from build123d import *

# Parameters (mm, degrees)
ESQUISSE1_R                  = 5.75
ESQUISSE1_R_2                = 1.6
BOSS_EXTRU_1_DEPTH           = 5
ESQUISSE2_R                  = 3
ENL_V_MAT_EXTRU_1_DEPTH      = 3
ENL_V_START                  = -3
ESQUISSE3_R                  = 5.75
ESQUISSE3_R_2                = 4.5
ENL_V_MAT_EXTRU_2_DEPTH      = 3
BOSS_EXTRU_2_DEPTH           = 2
R_P_TITION_CIRCULAIRE1_COUNT = 2
ESQUISSE5_R                  = 0.75
ENL_V_MAT_EXTRU_3_DEPTH      = 3
R_P_TITION_CIRCULAIRE2_COUNT = 2
BOSS_EXTRU_3_DEPTH           = 3
R_P_TITION_CIRCULAIRE3_COUNT = 28
ENL_V_START_2                = -1
ESQUISSE7_R                  = 3
ESQUISSE7_R_2                = 1.6
ENL_V_MAT_EXTRU_4_DEPTH      = 1
ESQUISSE8_R                  = 4.7
ESQUISSE8_R_2                = 3.4
ENL_V_MAT_EXTRU_5_DEPTH      = 1
WYTNIJ_WYCI_GNI_CIE1_DEPTH   = 10


with BuildPart() as part:
    # Esquisse1 → Boss.-Extru.1 (new body)
    with BuildSketch(Plane.XY):
        Circle(ESQUISSE1_R)
        Circle(ESQUISSE1_R_2, mode=Mode.SUBTRACT)
    extrude(amount=BOSS_EXTRU_1_DEPTH)

    # Esquisse2 → Enlèv. mat.-Extru.1 (cut)
    with BuildSketch(Plane.XY.offset(5)):
        Circle(ESQUISSE2_R)
    extrude(amount=-ENL_V_MAT_EXTRU_1_DEPTH, mode=Mode.SUBTRACT)

    # Esquisse3 → Enlèv. mat.-Extru.2 (cut)
    with BuildSketch(Plane.XY.offset(5).offset(ENL_V_START)):
        Circle(ESQUISSE3_R)
        Circle(ESQUISSE3_R_2, mode=Mode.SUBTRACT)
    extrude(amount=ENL_V_MAT_EXTRU_2_DEPTH, mode=Mode.SUBTRACT)

    # Esquisse4 → Boss.-Extru.2 (add)
    with BuildSketch(Plane(origin=(0, 0, 0), x_dir=(-1, 0, 0), z_dir=(0, 0, -1))):
        with BuildLine():
            Line((-4.3, 3.817394399), (-2.475852955, 16.846629695))
            ThreePointArc((-2.475852955, 16.846629695), (0, 19), (2.475852955, 16.846629695))
            Line((2.475852955, 16.846629695), (4.3, 3.817394399))
            ThreePointArc((4.3, 3.817394399), (0, 5.75), (-4.3, 3.817394399))
        make_face()
    boss_extru_2 = extrude(amount=-BOSS_EXTRU_2_DEPTH)

    # Répétition circulaire1: Boss.-Extru.2 ×2 about axis
    r_p_tition_circulaire1_axis = Axis((0, 0, 0), (0, 0, 1))
    for i in range(1, R_P_TITION_CIRCULAIRE1_COUNT):
        add(boss_extru_2.rotate(r_p_tition_circulaire1_axis, i * 360 / R_P_TITION_CIRCULAIRE1_COUNT))

    # Esquisse5 → Enlèv. mat.-Extru.3 (cut)
    with BuildSketch(Plane(origin=(0, 0, 0), x_dir=(-1, 0, 0), z_dir=(0, 0, -1))):
        with Locations((0, 7)):
            Circle(ESQUISSE5_R)
        with Locations((0, 10)):
            Circle(ESQUISSE5_R)
        with Locations((0, 13)):
            Circle(ESQUISSE5_R)
        with Locations((0, 16)):
            Circle(ESQUISSE5_R)
    enl_v_mat_extru_3 = extrude(amount=-ENL_V_MAT_EXTRU_3_DEPTH, mode=Mode.SUBTRACT)

    # Répétition circulaire2: Enlèv. mat.-Extru.3 ×2 about axis
    r_p_tition_circulaire2_axis = Axis((0, 0, 0), (0, 0, 1))
    for i in range(1, R_P_TITION_CIRCULAIRE2_COUNT):
        add(enl_v_mat_extru_3.rotate(r_p_tition_circulaire2_axis, i * 360 / R_P_TITION_CIRCULAIRE2_COUNT), mode=Mode.SUBTRACT)

    # Esquisse6 → Boss.-Extru.3 (add)
    with BuildSketch(Plane.XY.offset(5)):
        Polygon((-0.3, 3), (0, 2.7), (0.3, 3), align=None)
    boss_extru_3 = extrude(amount=-BOSS_EXTRU_3_DEPTH)

    # Répétition circulaire3: Boss.-Extru.3 ×28 about axis
    r_p_tition_circulaire3_axis = Axis((0, 0, 0), (0, 0, 1))
    for i in range(1, R_P_TITION_CIRCULAIRE3_COUNT):
        add(boss_extru_3.rotate(r_p_tition_circulaire3_axis, i * 360 / R_P_TITION_CIRCULAIRE3_COUNT))

    # Esquisse7 → Enlèv. mat.-Extru.4 (cut)
    with BuildSketch(Plane(origin=(0, 0, 0), x_dir=(-1, 0, 0), z_dir=(0, 0, -1)).offset(ENL_V_START_2)):
        Circle(ESQUISSE7_R)
        Circle(ESQUISSE7_R_2, mode=Mode.SUBTRACT)
    extrude(amount=ENL_V_MAT_EXTRU_4_DEPTH, mode=Mode.SUBTRACT)

    # Esquisse8 → Enlèv. mat.-Extru.5 (cut)
    with BuildSketch(Plane(origin=(0, 0, 0), x_dir=(-1, 0, 0), z_dir=(0, 0, -1))):
        Circle(ESQUISSE8_R)
        Circle(ESQUISSE8_R_2, mode=Mode.SUBTRACT)
    extrude(amount=-ENL_V_MAT_EXTRU_5_DEPTH, mode=Mode.SUBTRACT)

    # Szkic1 → Wytnij-wyciągnięcie1 (cut)
    with BuildSketch(Plane(origin=(0, 0, 0), x_dir=(-1, 0, 0), z_dir=(0, 0, -1))):
        with BuildLine():
            Line((3.959425115, -6.25), (-3.959425115, -6.25))
            Line((-3.959425115, -6.25), (-2.475852955, -16.846629695))
            ThreePointArc((-2.475852955, -16.846629695), (0, -19), (2.475852955, -16.846629695))
            Line((2.475852955, -16.846629695), (3.959425115, -6.25))
        make_face()
    extrude(amount=-WYTNIJ_WYCI_GNI_CIE1_DEPTH, mode=Mode.SUBTRACT)


solid = part.part
Work out the finished part from the listing and answer in its coordinate system (mm). A direction names the side the tool comes from. Give positions to 0.01 mm unless a question says otherwise; leave off trailing zeros. Loops run counter-clockwise (first coordinate to the right, second up) from the corner with the lowest first, then second, coordinate; pieces in that order, holes last. Notation, with made-up numbers: M 55,45.25 L 61,45.25 A25 cw 61,80.25 Z; hole C 5,35.25 d3. An arc over 180 degrees is marked long. Use CSV: the item, a comma, the result in double quotes.
1) Find section A-A on y = 10. Write down the section's boundary in (x, z), plus the area to 3 significant figures.
Answer:
outline,"M -3.43,0 L -0.75,0 L -0.75,2 L -3.43,2 Z; M 0.75,0 L 3.43,0 L 3.43,2 L 0.75,2 Z"
area,"10.7 mm^2"
2) Determine the mould class of faces 1 (the flat face through (0, -6.25, 1)), 2 (the flat face through (0, -3, 5)), 3 (the flat face through (1.3, -1.3, 2)) for opening direction Y: released by +Y, released by -Y, zero draft, split by the parting line, or undercut.
Answer:
face 1,"released by -Y"
face 2,"zero draft"
face 3,"undercut"
3) Consider L1, parallel to Y at x = 0, z = 1.35; L2, parallel to Z at x = -1, y = -4.75; L3, parallel to Z at x = -4, y = 1.5. Determine where each line is inside the solid, lowest interval first.
Answer:
L1,"-6.25 to -1.6, 1.6 to 6.25, 7.75 to 9.25, 10.75 to 12.25, 13.75 to 15.25, 16.75 to 19"
L2,"0 to 2"
L3,"1 to 5"
4) Find section B-B on y = 7. Write down the section's boundary in (x, z), plus the area to 3 significant figures.
Answer:
outline,"M -3.85,0 L -0.75,0 L -0.75,2 L -3.85,2 Z; M 0.75,0 L 3.85,0 L 3.85,2 L 0.75,2 Z"
area,"12.4 mm^2"
5) Given P1, Ø6, axis at x = 4, y = 13.5, coming from the +Z side; P2, Ø1.5, axis at x = 1, z = 3, coming from the -Y side; P3, Ø6.5, axis at x = -0.5, y = 1, coming from the -Z side; P4, Ø1.5, axis at y = -2.5, z = 2, coming from the +X side, each flat-ended and moving along its own axis, determine where each tip first touches the part or whether it passes through.
Answer:
P1,"z = 2"
P2,"y = -4.49"
P3,"z = 0"
P4,"x = 5.48"
6) Which of the six approach directions +Z, -Z, +X, -X, +Y, -Y give full straight-line access (tool end or side, diameter ignored) to faces 4 (the cylindrical face through (0.098, 13.744, 0.986)), 5 (the cylindrical face through (0.74, -3.32, 0.49))?
Answer:
face 4,"+Z, -Z"
face 5,"-Z"
